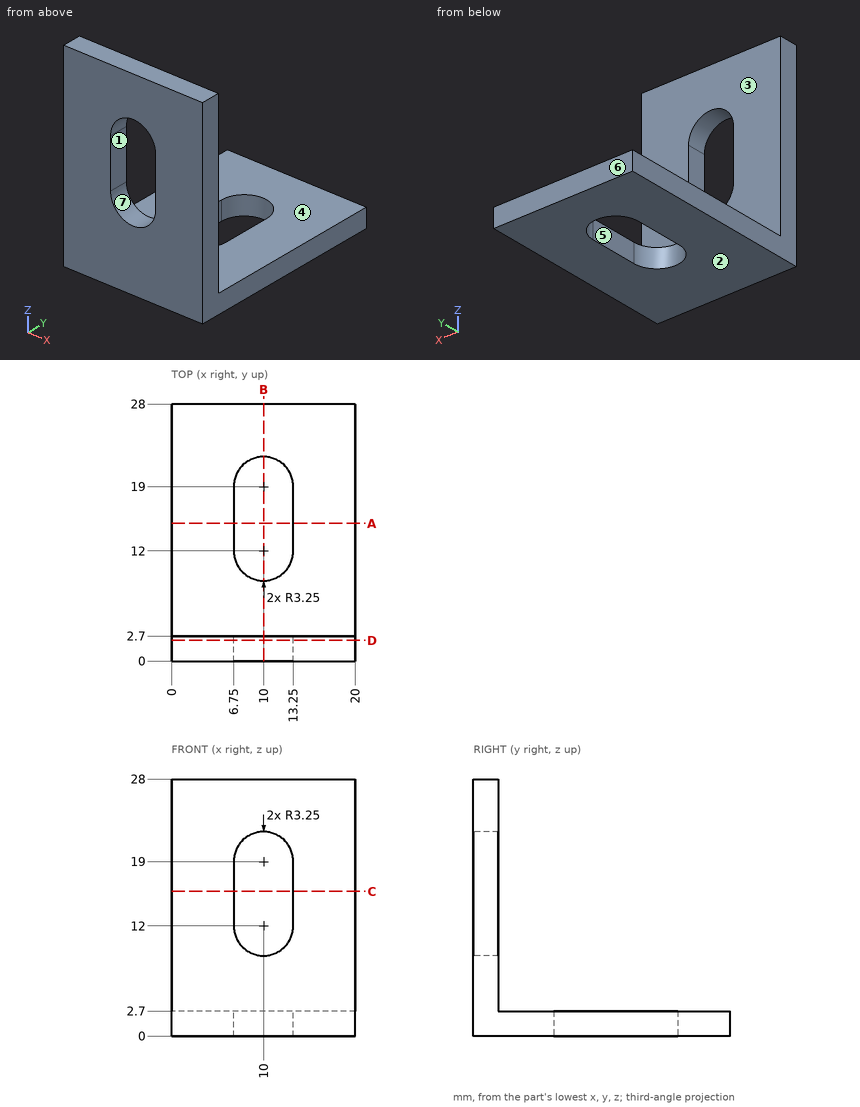
Source: three-view drawing plus pictorial views. Frame: mm from the lowest corner of the part. A direction names the side the tool comes from. Give positions to 0.01 mm unless a question says otherwise; leave off trailing zeros. Order: outer loops, then holes, each group sorted by start corner. A loop starts at its lowest first (then second) coordinate and runs counter-clockwise, first axis right, second up.
1. Mould query, pull axis Z, two halves, no side actions, for the marked faces 1, 2 and 3. Classes: released by +Z, released by -Z, zero draft, split by the parting line, or undercut.
Derived:
face 1: undercut
face 2: released by -Z
face 3: zero draft
2. Section D-D on y = 2.25. Return the cut outline in (x, z), and give its area (3 significant figures).
Derived:
outline: (0, 0) - (20, 0) - (20, 28) - (0, 28) - close; hole (6.75, 12) arc R3.25 ccw to (13.25, 12) - (13.25, 19) arc R3.25 ccw to (6.75, 19) - close
area: 481 mm2
3. Section A-A on y = 15. Return the cut outline in (x, z), and give its area (4 significant figures).
Derived:
outline: (0, 0) - (6.75, 0) - (6.75, 2.7) - (0, 2.7) - close; (13.25, 0) - (20, 0) - (20, 2.7) - (13.25, 2.7) - close
area: 36.45 mm2
4. Section B-B on x = 10. Return the cut outline in (y, z), and give its area (3 significant figures).
Derived:
outline: (0, 0) - (8.75, 0) - (8.75, 2.7) - (2.7, 2.7) - (2.7, 8.75) - (0, 8.75) - close; (0, 22.25) - (2.7, 22.25) - (2.7, 28) - (0, 28) - close; (22.25, 0) - (28, 0) - (28, 2.7) - (22.25, 2.7) - close
area: 71.0 mm2
5. Material intervals for L1, parallel to Z at x = 2, y = 19.25, sorted ascending.
Derived:
L1: z = 0 to 2.7
6. Reachability of the marked faces 4, 5, 6 and 7 from +Z, -Z, +X, -X, +Y, -Y: full face, straight path, thin tool, end or side. Return the list, or none.
Derived:
face 4: +Z, +X, -X, +Y
face 5: +Z, -Z
face 6: +Z, -Z, +X, -X, +Y
face 7: +Y, -Y
7. Pin query (flat end, axial travel): pin 1 (4 mm diameter, centred on x = 11.5, z = 9.5, fed in from +Y); pin 2 (10 mm diameter, centred on x = 14.5, y = 13, fed in from +Z). Return the tip coordinate at first contact, or that it passes through.
Derived:
pin 1: stops at y = 2.7
pin 2: stops at z = 2.7
